Read the model definition and answer for the solid it produces. Units are mm, in the model's axes. Face numbers are marked on the shaded views. Coordinates: 2 decimals unless noted, no trailing zeros. Loops run counter-clockwise (first coordinate to the right, second up) from the corner with the lowest first, then second, coordinate; pieces in that order, holes last. Notation, with made-up numbers: (73, -11) -> (77, -11) arc R9 cw to (77, 1) -> close; hole circle Ø2 at (-29, -10.5). An arc over 180 degrees is marked (long way). Answer as a JSON object with one key per item and string values. Group by question number.
Q1. Straight lines are drawn through the part: line 1 along X through (y, z) = (1.05, 0.25); line 2 along X through (y, z) = (0.2, 1.25); line 3 along Z through (x, y) = (21.5, -0.35). For each, find the intervals that lie inside material, in ascending order. Write a range as [from, to].
Q2. The part is cut by section B-B on x = 23.5. Write down the section's boundary in (y, z).
Q3. The part is cut by section C-C on y = -0.6. Write down the section's boundary in (x, z).
Q4. The part is cut by section A-A on z = 0. Write down the section's boundary in (x, y), and give its area (3 significant figures).
Q5. The part is cut by section D-D on z = -2.25. Write down the section's boundary in (x, y), and give its area (3 significant figures).
Q6. This flat-tipped pin is pushed along its axis until it touches: P1, Ø5, axis at x = -23.5, z = 0, coming from the -Y side. Where does it stop, or does it pass through?
Q7. Determine the mould class of the marked faces 1, 2 and 3 for opening direction X: released by +X, released by -X, zero draft, split by the parting line, or undercut.
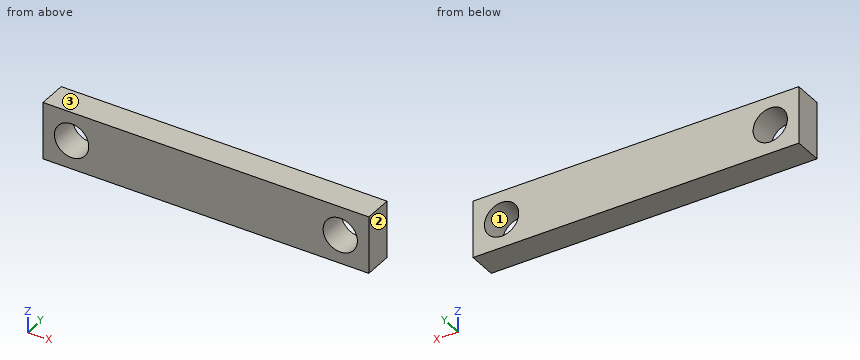
from build123d import *

# Parameters (mm, degrees)
SKETCH1_W           = 57
SKETCH1_H           = 10
SKETCH1_R           = 3
BOSS_EXTRUDE1_DEPTH = 2.5


with BuildPart() as part:
    # Sketch1 → Boss-Extrude1 (new, symmetric)
    with BuildSketch(Plane(origin=(0, 0, 0), x_dir=(1, 0, 0), z_dir=(0, 1, 0))):
        Rectangle(SKETCH1_W, SKETCH1_H)
        with Locations(Location((-23.5, 0, 0), (0, 0, 270))):
            Circle(SKETCH1_R, mode=Mode.SUBTRACT)
        with Locations(Location((23.5, 0, 0), (0, 0, 270))):
            Circle(SKETCH1_R, mode=Mode.SUBTRACT)
    extrude(amount=BOSS_EXTRUDE1_DEPTH, both=True)


solid = part.part
Final values:
{
 "1": {"line 1": "x = [-28.5, -26.49], [-20.51, 20.51], [26.49, 28.5]", "line 2": "x = [-28.5, -26.23], [-20.77, 20.77], [26.23, 28.5]", "line 3": "z = [-5, -2.24], [2.24, 5]"},
 "2": {"outline": "(-2.5, -5) -> (2.5, -5) -> (2.5, -3) -> (-2.5, -3) -> close; (-2.5, 3) -> (2.5, 3) -> (2.5, 5) -> (-2.5, 5) -> close"},
 "3": {"outline": "(-28.5, -5) -> (28.5, -5) -> (28.5, 5) -> (-28.5, 5) -> close; hole circle Ø6 at (-23.5, 0); hole circle Ø6 at (23.5, 0)"},
 "4": {"outline": "(-28.5, -2.5) -> (-26.5, -2.5) -> (-26.5, 2.5) -> (-28.5, 2.5) -> close; (-20.5, -2.5) -> (20.5, -2.5) -> (20.5, 2.5) -> (-20.5, 2.5) -> close; (26.5, -2.5) -> (28.5, -2.5) -> (28.5, 2.5) -> (26.5, 2.5) -> close", "area": "225 mm2"},
 "5": {"outline": "(-28.5, -2.5) -> (-25.48, -2.5) -> (-25.48, 2.5) -> (-28.5, 2.5) -> close; (-21.52, -2.5) -> (21.52, -2.5) -> (21.52, 2.5) -> (-21.52, 2.5) -> close; (25.48, -2.5) -> (28.5, -2.5) -> (28.5, 2.5) -> (25.48, 2.5) -> close", "area": "245 mm2"},
 "6": {"P1": "passes through"},
 "7": {"face 1": "undercut", "face 2": "released by +X", "face 3": "zero draft"}
}
